Autodesk Inventor part; units mm, degrees
ref_plane "YZ Plane" through (0, 0, 0) normal (1, 0, 0) x (0, 1, 0)
ref_plane "XZ Plane" through (0, 0, 0) normal (0, 1, 0) x (-1, 0, 0)
ref_plane "XY Plane" through (0, 0, 0) normal (0, 0, 1) x (1, 0, 0)
sketch "Sketch1" plane through (0, 0, 0) normal (0, 1, 0) x (-1, 0, 0)
  line L0 (49.7782, 121.4529) -> (24.3782, 121.4529)
  line L1 (24.3782, 121.4529) -> (24.3782, -488.1471)
  line L2 (24.3782, -488.1471) -> (49.7782, -488.1471)
  line L3 (49.7782, -488.1471) -> (49.7782, 121.4529)
  point P0 (0, 0)
  dimension "d0" = 25.4
  dimension "d1" = 609.6
extrude "Extrusion1" add sketch "Sketch1" along normal blind 25.4
sketch "Sketch2" plane through (-49.7782, 0, 121.4529) normal (0, 0, 1) x (1, 0, 0)
  line L0 (0, 25.4) -> (25.4, 25.4)
  line L1 (25.4, 25.4) -> (25.4, 0)
  line L2 (25.4, 0) -> (0, 0)
  line L3 (0, 0) -> (0, 25.4)
  line L4 (3.175, 22.225) -> (22.225, 22.225)
  line L5 (22.225, 22.225) -> (22.225, 3.175)
  line L6 (22.225, 3.175) -> (3.175, 3.175)
  line L7 (3.175, 3.175) -> (3.175, 22.225)
  point P0 (49.7782, 0)
  dimension "d5" = 3.175
  dimension "d6" = 3.175
  dimension "d7" = 3.175
  dimension "d8" = 3.175
extrude "Extrusion2" cut sketch "Sketch2" against normal blind 508 contours L4 L5 L6 L7
sketch "Sketch3" plane through (-24.3782, 0, 121.4529) normal (1, 0, 0) x (0, 0, -1)
  circle A0 centre (241.3, 19.05) radius 3.175
  circle A1 centre (241.3, 6.35) radius 3.175
  line L0 (0, 25.4) -> (609.6, 25.4)
  line L1 (0, 0) -> (0, 25.4)
  line L2 (304.8, 25.4) -> (304.8, 0) construction
  circle A2 centre (368.3, 19.05) radius 3.175
  circle A3 centre (368.3, 6.35) radius 3.175
  point P0 (121.4529, 0)
  dimension "d11" = 6.35
  dimension "d12" = 6.35
  dimension "d14" = 12.7
  dimension "d15" = 6.35
  dimension "d26" = 304.8
  dimension "d27" = 63.5
  dimension "d28" = 63.5
extrude "Extrusion3" cut sketch "Sketch3" against normal blind 12.7
sketch "Sketch4" plane through (-24.3782, 0, 121.4529) normal (1, 0, 0) x (0, 0, -1)
  line L0 (0, 25.4) -> (609.6, 25.4) construction
  line L1 (304.8, 25.4) -> (304.8, 0) construction
  line L2 (0, 0) -> (0, 25.4) construction
  line L3 (120.65, 25.4) -> (120.65, 0) construction
  circle A0 centre (120.65, 12.7) radius 3.175
  circle A1 centre (488.95, 12.7) radius 3.175
  point P0 (121.4529, 0)
  dimension "d20" = 304.8
  dimension "d21" = 184.15
  dimension "d22" = 6.35
  dimension "d23" = 12.7
extrude "Extrusion4" cut sketch "Sketch4" against normal blind 25.4
sketch "Sketch6" plane through (-24.3782, 0, 121.4529) normal (1, 0, 0) x (0, 0, -1)
  line L0 (0, 0) -> (609.6, 0)
  line L1 (304.8, 0) -> (304.8, 25.4)
  line L2 (0, 25.4) -> (609.6, 25.4)
  line L3 (0, 0) -> (0, 25.4)
  circle A0 centre (50.8, 12.7) radius 3.175
  circle A1 centre (558.8, 12.7) radius 3.175
  point P0 (121.4529, 0)
  dimension "d29" = 304.8
  dimension "d30" = 6.35
  dimension "d31" = 12.7
  dimension "d32" = 254
extrude "Extrusion5" cut sketch "Sketch6" against normal blind 25.4 contours A0 | A1
properties part number "clawBase"
Can you work these out from the model? Positions are in its coordinate system, mm. A direction names the side the tool comes from. Give positions to 0.01 mm unless a question says otherwise; leave off trailing zeros. Order: outer loops, then holes, each group sorted by start corner. A loop starts at its lowest first (then second) coordinate and runs counter-clockwise, first axis right, second up. Notation, with made-up numbers: (-6.75, 26) - (51.25, 26) arc R19 ccw to (51.25, 55) - close; hole circle Ø3 at (47.5, 74). An arc over 180 degrees is marked (long way). Write each question's results on one line, items separated by ' | '.
1) I'm going to push a flat-ended pin straight in: pin 1 Ø12 at (x, y) = (-45, 21.5) entering from +Z. Where does the tip first touch, or does it pass through?
Final values:
pin 1: stops at z = 121.45
2) Please list where these lines run through material, in increasing order: line 1 along Z through (x, y) = (-25.95, 19.05); line 2 along Y through (x, z) = (-40.5, 49) (3 decimals); line 3 along X through (y, z) = (14.75, -222.5). Write a range as [from, to].
Final values:
line 1: z = [-488.15, -250.02], [-243.67, -123.02], [-116.67, 121.45] | line 2: y = [0, 3.175], [22.225, 25.4] | line 3: x = [-49.78, -46.6], [-27.55, -24.38]
3) Suppose I cut it at B-B, the plane z = -377. Write out the boundary of the cut face in (x, y) (3 decimals), then the cut area to 3 significant figures.
Final values:
outline: (-49.778, 0) - (-24.378, 0) - (-24.378, 25.4) - (-49.778, 25.4) - close; hole (-46.603, 3.175) - (-27.553, 3.175) - (-27.553, 22.225) - (-46.603, 22.225) - close | area: 282 mm^2
4) On a 3-axis mill with a long thin cutter (end or side, diameter ignored), from which of +Z, -Z, +X, -X, +Y, -Y can I reach the whole of each face in a straight line? I mean faces 1 (the face through (-46.603, 13, -129)), 2 (the face through (-37, 25.4, -179)). Say none if no direction works.
Final values:
face 1: +Z | face 2: +Z, -Z, +X, -X, +Y
5) Suppose I cut it at A-A, the plane x = -36. Write out the boundary of the cut face in (y, z) (3 decimals), then the cut area to 3 significant figures.
Final values:
outline: (0, -488.147) - (25.4, -488.147) - (25.4, 121.453) - (22.225, 121.453) - (22.225, -386.547) - (3.175, -386.547) - (3.175, 121.453) - (0, 121.453) - close; hole circle Ø6.35 at (12.7, -437.347) | area: 5,770 mm^2
